Read the model definition and answer for the solid it produces. Units are mm, in the model's axes. A direction names the side the tool comes from. Coordinates: 2 decimals unless noted, no trailing zeros. One line per question, with ' | ' between items. Start each with the question number.
1) A tool of negligible diameter and unlimited length cuts with its end or side. For faces 1 (the face through (-27, -107.5, -3)), 2 (the face through (-6, -108, -4)), from which of +Z, -Z, +X, -X, +Y, -Y can it reach the whole face along a straight path? Write none if from no direction.
2) Given P1, Ø2, axis at x = 7.5, y = -114, coming from the +Z side; P2, Ø1, axis at y = -106, z = -3, coming from the +X side; P3, Ø13, axis at x = 0, y = -108.5, coming from the +Z side; P4, Ø0.6, axis at y = -108, z = -3, coming from the -X side, each flat-ended and moving along its own axis, determine where each tip first touches the part or whether it passes through.
3) Consider probe 1 along Z at (x, y) = (15, -126); probe 2 along Y at (x, z) = (0, -2.2); probe 3 along X at (y, z) = (-111.5, -1.4). Determine where each line is inside the solid, lowest interval first.
4) The mould has two halves that part along Y. Classify faces 3 (the face through (-0.78, -102.55, -1.75)), 4 (the face through (-4, -110, 0)), 5 (the face through (-27, -109.5, -3)): +Y half, -Y half, draft (parallel to the pull), parting line (faces both ways), or undercut.
from build123d import *

# Parameters (mm, degrees)
SKETCH1_R           = 6
BOSS_EXTRUDE1_DEPTH = 2
SKETCH2_R           = 28.8
BOSS_EXTRUDE2_DEPTH = 2
SKETCH3_R           = 4
CUT_EXTRUDE1_DEPTH  = 141.3450391
FILLET1_R           = 1.5
FILLET2_R           = 1
SKETCH4_W           = 6
SKETCH4_H           = 2
CUT_EXTRUDE2_DEPTH  = 141.345039121


with BuildPart() as part:
    # Sketch1 → Boss-Extrude1 (new body)
    with BuildSketch(Plane.XY):
        with Locations((0, -108.5)):
            Circle(SKETCH1_R)
    extrude(amount=-BOSS_EXTRUDE1_DEPTH)

    # Sketch2 → Boss-Extrude2 (add)
    with BuildSketch(Plane(origin=(0, 0, -2), x_dir=(-1, 0, 0), z_dir=(0, 0, -1))):
        with Locations((0, -108.5)):
            Circle(SKETCH2_R)
    extrude(amount=BOSS_EXTRUDE2_DEPTH)

    # Sketch3 → Cut-Extrude1 (cut, through all)
    with BuildSketch(Plane.XY):
        with Locations((0, -108.5)):
            Circle(SKETCH3_R)
    extrude(amount=-CUT_EXTRUDE1_DEPTH, mode=Mode.SUBTRACT)

    # Fillet1
    fillet1_edges = [part.edges().sort_by_distance(p)[0] for p in [
        (-6, -108.5, 0),
    ]]
    fillet(fillet1_edges, radius=FILLET1_R)

    # Fillet2
    fillet2_edges = [part.edges().sort_by_distance(p)[0] for p in [
        (28.8, -108.5, -2),
        (28.8, -108.5, -4),
    ]]
    fillet(fillet2_edges, radius=FILLET2_R - 0.0001)  # a hair under: the kernel refuses the full size

    # Sketch4 → Cut-Extrude2 (cut, through all)
    with BuildSketch(Plane.XY):
        with Locations((-28.782633653, -108.5)):
            Rectangle(SKETCH4_W, SKETCH4_H)
    extrude(amount=-CUT_EXTRUDE2_DEPTH, mode=Mode.SUBTRACT)


solid = part.part
Report:
1) face 1: +Z, -Z, -X | face 2: -Z, +X, -X, +Y, -Y
2) P1: stops at z = -2 | P2: stops at x = 28.73 | P3: stops at z = 0 | P4: stops at x = -25.78
3) probe 1: z = -4 to -2 | probe 2: y = -136.9 to -112.5, -104.5 to -80.1 | probe 3: x = -5.19 to -2.65, 2.65 to 5.19
4) face 3: parting line | face 4: draft | face 5: undercut
